```python
from build123d import *
from build123d.topology import SkipClean

# Parameters (mm, degrees)
BOSS_EXTRUDE1_DEPTH   = 3
BOSS_EXTRUDE1_2_DEPTH = 3
BOSS_EXTRUDE2_DEPTH   = 20.7
BOSS_EXTRUDE3_DEPTH   = 3
BOSS_EXTRUDE4_START   = 15
BOSS_EXTRUDE4_DEPTH   = 15


with BuildPart() as part:
    # Sketch1 → Boss-Extrude1 (new body)
    with BuildSketch(Plane(origin=(0, 0, 0), x_dir=(1, 0, 0), z_dir=(0, 1, 0))):
        with BuildLine():
            Line((-126.934037988, 12), (126.934037988, 12))
            ThreePointArc((126.934037988, 12), (0, 127.5), (-126.934037988, 12))
        make_face()
    extrude(amount=BOSS_EXTRUDE1_DEPTH)



with BuildPart() as body_2:
    # Sketch1 → Boss-Extrude1 2 (new body)
    with BuildSketch(Plane(origin=(0, 0, 0), x_dir=(1, 0, 0), z_dir=(0, 1, 0))):
        with BuildLine():
            Line((-126.223016918, -18), (126.223016918, -18))
            ThreePointArc((126.223016918, -18), (0, -127.5), (-126.223016918, -18))
        make_face()
    extrude(amount=BOSS_EXTRUDE1_2_DEPTH)


with BuildPart() as part_1:
    with SkipClean():  # the faces are left unmerged after this step: merging them gives an invalid solid
        add(part.part)

        add(body_2.part)  # Boss-Extrude2 merges body 2
        # Sketch5 → Boss-Extrude2 (add)
        with BuildSketch(Plane(origin=(0, 3, 0), x_dir=(1, 0, 0), z_dir=(0, 1, 0))):
            with BuildLine():
                Line((-126.614572621, 15), (126.614572621, 15))
                ThreePointArc((126.614572621, 15), (126.783179032, 13.50094495), (126.934037988, 12))
                Line((126.934037988, 12), (-126.934037988, 12))
                ThreePointArc((-126.934037988, 12), (-126.783179032, 13.50094495), (-126.614572621, 15))
            make_face()
            with BuildLine():
                Line((-125.758697512, -21), (125.758697512, -21))
                ThreePointArc((125.758697512, -21), (125.999786118, -19.501381954), (126.223016918, -18))
                Line((126.223016918, -18), (-126.223016918, -18))
                ThreePointArc((-126.223016918, -18), (-125.999786118, -19.501381954), (-125.758697512, -21))
            make_face()
        extrude(amount=BOSS_EXTRUDE2_DEPTH)

    # Sketch6 → Boss-Extrude3 (add)
    with BuildSketch(Plane(origin=(0, 23.7, 0), x_dir=(1, 0, 0), z_dir=(0, 1, 0))):
        with BuildLine():
            Line((-126.614572621, 15), (126.614572621, 15))
            ThreePointArc((126.614572621, 15), (127.463982636, -3.030368055), (125.758697512, -21))
            Line((125.758697512, -21), (-125.758697512, -21))
            ThreePointArc((-125.758697512, -21), (-127.463982636, -3.030368055), (-126.614572621, 15))
        make_face()
    extrude(amount=BOSS_EXTRUDE3_DEPTH)

    # Sketch7 → Boss-Extrude4 (add)
    with BuildSketch(Plane.XZ.offset(BOSS_EXTRUDE4_START)):
        with BuildLine():
            Line((-126.934037988, -12), (-123.977391141, -12))
            ThreePointArc((-123.977391141, -12), (0, -124.55678831), (123.977391141, -12))
            Line((123.977391141, -12), (126.934037988, -12))
            ThreePointArc((126.934037988, -12), (0, -127.5), (-126.934037988, -12))
        make_face()
        with BuildLine():
            Line((123.191923437, 18), (126.223016918, 18))
            ThreePointArc((126.223016918, 18), (0, 127.5), (-126.223016918, 18))
            Line((-126.223016918, 18), (-123.191923437, 18))
            ThreePointArc((-123.191923437, 18), (0, 124.5), (123.191923437, 18))
        make_face()
    extrude(amount=-BOSS_EXTRUDE4_DEPTH)


solid = part_1.part
```
CAD build for the part. Positions are in the model's coordinates, mm. A direction names the side the tool comes from. Round coordinates to 2 decimals unless told otherwise and drop trailing zeros. Order: outer loops, then holes, each group sorted by start corner. A loop starts at its lowest first (then second) coordinate and runs counter-clockwise, first axis right, second up.
Item 1: Saw through at D-D on z = 39. Write the cut outline in (x, y), then the cut area to 3 significant figures.
Item 2: Saw through at B-B on y = 8.5. Write the cut outline in (x, z).
Item 3: Saw through at C-C on x = -82. Write the cut outline in (y, z), then the cut area to 3 significant figures.
Item 4: Tool access for faces 3 (the face through (2, 0, 59)), 4 (the face through (2, 3, 62)), 5 (the face through (-2, 3, -60)), 6 (the face through (-2, 13, -12)), 7 (the face through (10, -15, -125)): list every direction of +Z, -Z, +X, -X, +Y, -Y with a clear straight run to the whole face (end or side of a thin tool).
Item 5: Saw through at A-A on y = -8.5. Write the cut outline in (x, z), then the cut area to 3 significant figures.
Item 6: Pin check, flat tips, straight feed: pin 1 (4 mm diameter, centred on x = -85, y = 14, fed in from +Z); pin 2 (3 mm diameter, centred on x = 36.5, y = -9.5, fed in from +Z); pin 3 (6 mm diameter, centred on y = 3.5, z = -75, fed in from -X). Stop position of each tip, or through.
Item 7: Mould opens along X. For faces 1 (the face through (-2, 0, -57)), 2 (the face through (-10, -15, 126)) say: pulls with the +X half, pulls with the -X half, needs draft (parallel to the pull), parting line crosses it, or undercut.
Item 8: Probe line 1 along Z through (x, y) = (9, 23.5); line 2 along Y through (x, z) = (75.5, 83); line 3 along Y through (x, z) = (57.5, 13.5). List the from-to ranges inside material, lowest first.
Reported:
1. outline: (-121.39, -15) - (-118.23, -15) - (-118.23, 0) - (118.23, 0) - (118.23, -15) - (121.39, -15) - (121.39, 3) - (-121.39, 3) - close
1. area: 823 mm2
2. outline: (-126.93, -12) arc R127.5 ccw to (-126.61, -15) - (126.61, -15) arc R127.5 ccw to (126.93, -12) - close; (-126.22, 18) - (126.22, 18) arc R127.5 ccw to (125.76, 21) - (-125.76, 21) arc R127.5 ccw to start
3. outline: (-15, -97.63) - (3, -97.63) - (3, -15) - (26.7, -15) - (26.7, 21) - (3, 21) - (3, 97.63) - (-15, 97.63) - (-15, 93.68) - (0, 93.68) - (0, 18) - (23.7, 18) - (23.7, -12) - (0, -12) - (0, -93.76) - (-15, -93.76) - close
3. area: 845 mm2
4. face 3: -Y
4. face 4: +Z, +X, -X, +Y
4. face 5: -Z, +X, -X, +Y
4. face 6: +X, -X, -Y
4. face 7: +Z, -Z, +X, -X, -Y
5. outline: (-126.93, -12) arc R127.5 ccw to (126.93, -12) - (123.98, -12) arc R124.56 cw to (-123.98, -12) - close; (-126.22, 18) - (-123.19, 18) arc R124.5 cw to (123.19, 18) - (126.22, 18) arc R127.5 ccw to start
5. area: 2,170 mm2
6. pin 1: stops at z = 21
6. pin 2: stops at z = 122.6
6. pin 3: stops at x = -105.2
7. face 1: undercut
7. face 2: needs draft
8. line 1: z = -15 to -12, 18 to 21
8. line 2: y = 0 to 3
8. line 3: y = 23.7 to 26.7
